Verification items for the finished model (mm, model axes). Face numbers are marked on the shaded views. A direction names the side the tool comes from. Coordinates: 2 decimals unless noted, no trailing zeros. Order: outer loops, then holes, each group sorted by start corner. A loop starts at its lowest first (then second) coordinate and runs counter-clockwise, first axis right, second up. Notation, with made-up numbers: (-3, -3) - (34, -3) arc R17 cw to (34, 5) - close; hole circle Ø6 at (71, 2). An arc over 180 degrees is marked (long way). Answer as CSV lines item,"result". Start each with the question number.
1. Section check A-A (x = 2). Record the cut outline in (y, z), and give its area (3 significant figures).
2. Set-up check for the marked faces 4 and 5: record each of +Z, -Z, +X, -X, +Y, -Y from which the full face is reachable in a straight line by a thin tool's end or side.
3. Section check B-B (z = -26). Record the cut outline in (x, y).
4. Section check D-D (x = -9.5). Record the cut outline in (y, z), and give its area (3 significant figures).
5. Mould release check, pull along Z, two halves, no side actions. Record for the marked faces 1, 2 and 3: pulls with the +Z half, pulls with the -Z half, needs draft (parallel to the pull), parting line crosses it, or undercut.
6. Section check C-C (z = -48.5). Record the cut outline in (x, y).
7. Go/stop test with flat-tipped pins: pin 1 (0.6 mm diameter, centred on x = -30, y = -8.5, fed in from +Z); pin 2 (2 mm diameter, centred on x = -12.5, y = -6, fed in from +Z); pin 3 (10 mm diameter, centred on x = -31, z = -13, fed in from -Y). Record where each tip stops, or that it passes through.
8. Material ranges on L1, parallel to Y at x = -6, z = -35; L2, parallel to Y at x = 0, z = -6.5; L3, parallel to Z at x = -2, y = -0.5, recorded low to high. Write a range as [from, to].
from build123d import *

# Parameters (mm, degrees)
F0_W      = 61.1160316085
F0_H      = 104.14
F1_DEPTH  = 8.128
F2_R      = 5.08
F4_W      = 9.1636627913
F4_H      = 2.2909147665
F4_R      = 1.8469945904
F5_DEPTH  = 0.254
F6_W      = 23.6879978329
F6_H      = 2.015999984
F7_DEPTH  = 0.254
F3_W      = 53.0287652906
F3_H      = 38.1
F8_DEPTH  = 0.762
F3_R      = 7.62
F9_DEPTH  = 0.254
F3_R_2    = 17.78
F10_DEPTH = 0.254


# Not quite as in the source:
# - the program builds the solid bodies; features that only make, move or delete a surface that nothing else refers to are left out


with BuildPart() as f1:
    # F0 (on Front) → F1 (new body)
    with BuildSketch(Plane.XZ):
        with Locations((-19.607455004, -3.8571991026)):
            Rectangle(F0_W, F0_H)
    extrude(amount=F1_DEPTH)

    # F2
    f2_edges = [f1.edges().sort_by_distance(p)[0] for p in [
        (10.950561, -4.064, 48.212801),
        (-50.165471, -4.064, 48.212801),
        (10.950561, -4.064, -55.927199),
        (-50.165471, -4.064, -55.927199),
    ]]
    fillet(f2_edges, radius=F2_R)

    # F4 (on face) → F5 (join)
    with BuildSketch(Plane.XY.offset(48.2128008974)):
        with Locations((-37.6597046852, -3.8777994923)):
            Rectangle(F4_W, F4_H)
        with Locations((-2.1505255718, -3.8777994923)):
            Circle(F4_R)
    extrude(amount=F5_DEPTH)

    # F6 (on face) → F7 (join)
    with BuildSketch(Plane(origin=(0, 0, -55.9271991026), x_dir=(1, 0, 0), z_dir=(0, 0, -1))):
        with Locations((-19.78199929, 4.4100000523)):
            Rectangle(F6_W, F6_H)
    extrude(amount=F7_DEPTH)

    # F3 (on face) → F8 (join)
    with BuildSketch(Plane.XZ.offset(8.128)):
        with Locations((-19.607455004, 24.4255777958)):
            Rectangle(F3_W, F3_H)
    extrude(amount=F8_DEPTH)

    # F3 (on face) → F9 (join)
    with BuildSketch(Plane.XZ.offset(8.128)):
        with Locations((-19.607455004, -24.6234625244)):
            Circle(F3_R)
    extrude(amount=F9_DEPTH)

    # F3 (on face) → F10 (join)
    with BuildSketch(Plane.XZ.offset(8.128)):
        with Locations((-19.607455004, -24.6234625244)):
            Circle(F3_R_2)
        with Locations((-19.607455004, -24.6234625244)):
            Circle(F3_R, mode=Mode.SUBTRACT)
    extrude(amount=F10_DEPTH)


solid = f1.part
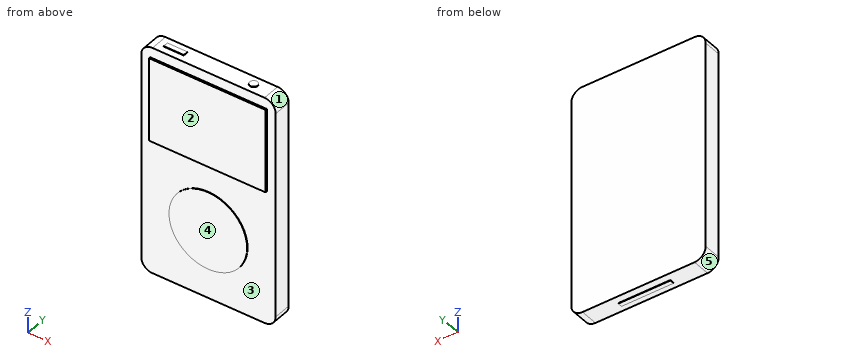
Evaluation:
1,outline,"(-8.89, 5.38) - (-8.13, 5.38) - (-8.13, -55.93) - (0, -55.93) - (0, 48.21) - (-8.13, 48.21) - (-8.13, 43.48) - (-8.89, 43.48) - close"
1,area,"875 mm²"
2,face 4,"-Z, +X, -X, -Y"
2,face 5,"-Z, -X, +Y, -Y"
3,outline,"(-50.17, -8.13) - (-37.33, -8.13) - (-37.33, -8.38) - (-1.88, -8.38) - (-1.88, -8.13) - (10.95, -8.13) - (10.95, 0) - (-50.17, 0) - close"
4,outline,"(-8.89, 5.38) - (-8.13, 5.38) - (-8.13, -10) - (-8.38, -10) - (-8.38, -39.25) - (-8.13, -39.25) - (-8.13, -55.93) - (-5.42, -55.93) - (-5.42, -56.18) - (-3.4, -56.18) - (-3.4, -55.93) - (0, -55.93) - (0, 48.21) - (-8.13, 48.21) - (-8.13, 43.48) - (-8.89, 43.48) - close"
4,area,"883 mm²"
5,face 1,"pulls with the +Z half"
5,face 2,"needs draft"
5,face 3,"undercut"
6,outline,"(-50.17, -8.13) - (10.95, -8.13) - (10.95, 0) - (-50.17, 0) - close"
7,pin 1,"stops at z = 43.48"
7,pin 2,"stops at z = 48.21"
7,pin 3,"stops at y = -8.38"
8,L1,"y = [-8.38, 0]"
8,L2,"y = [-8.13, 0]"
8,L3,"z = [-55.93, 48.21]"
